from build123d import *

# Parameters (mm, degrees)
F4_DEPTH  = 25.4
F5_W      = 46.6010663658
F5_H      = 39.7627335042
F6_DEPTH  = 25.4
F8_W      = 68.0729933083
F8_H      = 50.7683739997
F9_DEPTH  = 25.4
F11_W     = 45.6217722967
F11_H     = 58.1790879369
F12_DEPTH = 25.4


with BuildPart() as f4:
    # F0 (on Top) → F4 (new body)
    with BuildSketch(Plane.XY):
        Polygon((0, -12.7), (0, 0), (-7.3323484187, 0), align=None)
        Polygon((-7.3323484187, 0), (0, 0), (0, 12.7), (-10.9985226281, 6.35), align=None)
        Polygon((-21.9970452561, 0), (0, -12.7), (-7.3323484187, 0), align=None)
        Polygon((-21.9970452561, 0), (-7.3323484187, 0), (-10.9985226281, 6.35), align=None)
    extrude(amount=F4_DEPTH)

    # F5 (on 3pt) → F6 (cut)
    with BuildSketch(Plane(origin=(0, 0, 0), x_dir=(0, -1, 0), z_dir=(-0.9428090416, 0, -0.3333333333))):
        with Locations((-4.0135839954, 15.0211239234)):
            Rectangle(F5_W, F5_H)
    extrude(amount=-F6_DEPTH, mode=Mode.SUBTRACT)

    # F8 (on 3pt) → F9 (cut)
    with BuildSketch(Plane(origin=(-4.8882322791, -8.4666666667, 3.4565021926), x_dir=(0.8819171037, -0.4364357805, 0.1781741613), z_dir=(-0.4714045208, -0.8164965809, 0.3333333333))):
        with Locations((0.508910045, 15.6671002042)):
            Rectangle(F8_W, F8_H)
    extrude(amount=F9_DEPTH, mode=Mode.SUBTRACT)

    # F11 (on 3pt) → F12 (cut)
    with BuildSketch(Plane(origin=(-4.8882322791, 8.4666666667, 3.4565021926), x_dir=(-0.8819171037, -0.4364357805, -0.1781741613), z_dir=(-0.4714045208, 0.8164965809, 0.3333333333))):
        with Locations((11.0377906822, 16.6354514658)):
            Rectangle(F11_W, F11_H)
    extrude(amount=F12_DEPTH, mode=Mode.SUBTRACT)


solid = f4.part
Input: part model. Units: mm. Frame: model coordinates. Give positions to 0.01 mm unless a question says otherwise; leave off trailing zeros. Order: outer loops, then holes, each group sorted by start corner. A loop starts at its lowest first (then second) coordinate and runs counter-clockwise, first axis right, second up. Notation, with made-up numbers: M 67.25,51 L 99.25,51 A14 cw 99.25,74 Z; hole C -21,9 d1. An arc over 180 degrees is marked long. Answer as a JSON object with one key per item and string values.
1. Cut plane D-D, the plane x = -6.5. Output: boundary loops of the cut face in (y, z), and give its area (3 significant figures).
Result sheet:
{"outline": "M -8.95,0 L 8.95,0 L 1.44,18.38 L -1.44,18.38 Z", "area": "191 mm²"}
2. First-contact query: P1, Ø1.5, axis at x = -7.5, z = 11, coming from the -Y side; P2, Ø4, axis at y = -9.5, z = 3.5, coming from the +X side; P3, Ø4, axis at x = -8.5, z = 17, coming from the -Y side; P4, Ø6, axis at x = -17.5, y = -9.5, coming from the +Z side. Flat tips, straight axial feed; report the tip coordinate or a pass-through.
Result sheet:
{"P1": "y = -4.41", "P2": "x = -0.53", "P3": "y = -2.27", "P4": "through"}
3. Cut plane C-C, the plane x = -2. Output: boundary loops of the cut face in (y, z).
Result sheet:
{"outline": "M -11.55,0 L 11.55,0 L 9.24,5.66 L -9.24,5.66 Z"}
4. Cut plane A-A, the plane z = 10.25. Output: boundary loops of the cut face in (x, y), and give its area (3 significant figures).
Result sheet:
{"outline": "M -14.75,0 L -3.62,-6.42 L -3.62,6.42 Z", "area": "71.5 mm²"}
5. Cut plane B-B, the plane x = -12. Output: boundary loops of the cut face in (y, z), and give its area (3 significant figures).
Result sheet:
{"outline": "M -5.77,0 L 5.77,0 L 0,14.14 Z", "area": "81.6 mm²"}
6. Ray query, line 1 (Z direction, x = -8.5, y = 5.5); line 2 (Y direction, x = -8.25, z = 3); line 3 (Y direction, x = -11.75, z = 9.5). Return the intervals inside material, ascending. Write a range as [from, to].
Result sheet:
{"line 1": "[0, 5.62]", "line 2": "[-6.71, 6.71]", "line 3": "[-2.04, 2.04]"}
